Design review of the part built by this model. Coordinates are the model's own, in mm. A direction names the side the tool comes from. Coordinates: 2 decimals unless noted, no trailing zeros. Loops run counter-clockwise (first coordinate to the right, second up) from the corner with the lowest first, then second, coordinate; pieces in that order, holes last. Notation, with made-up numbers: (33, -2) - (90, -2) arc R34 ccw to (90, 35) - close; hole circle Ø10 at (-4.5, 35). An arc over 180 degrees is marked (long way). Use one line per item in the form item = value. Start each with the question number.
(1) For L1, parallel to Z at x = 0, y = -20; L2, parallel to Y at x = 31, z = 137.5; L3, parallel to Z at x = 0, y = -113.5, list the stretches that pass through material, from the lowest coordinate up.
(2) Clearance check with flat-ended pins moving along their axes: pin 1 Ø1.5 at (x, z) = (-20.5, 93.5) entering from +Y; pin 2 Ø5 at (x, y) = (36.5, -26.5) entering from +Z; pin 3 Ø10 at (y, z) = (-75, -24.5) entering from -X; pin 4 Ø20.5 at (y, z) = (-119, 65) entering from +X. State where each tip first meets the part, or that it passes through.
(3) Add section D-D (z = 34.5). State the section outline as (x, y) points.
(4) Tool access review of faces 1 (the face through (-9.97, -62.61, -44.9)), 2 (the face through (-45.142, -13, 59)), 3 (the face through (-0.993, -12.522, 155.356)): name each direction out of +Z, -Z, +X, -X, +Y, -Y from which nothing blocks a thin tool from reaching the whole face with its end or side.
(5) The part is to be moulded in two halves that separate along Z. For faces 4 (the face through (-3.374, -64.389, -15.192)), 5 (the face through (45.862, -114, 56)), 6 (the face through (3.25, -114.12, 119.93)), 7 (the face through (1.007, -114.478, 156.372)), say which applies: pulls with the +Z half, pulls with the -Z half, needs draft (parallel to the pull), parting line crosses it, or undercut.
(6) Add section A-A (x = 0). State the section outline as (y, z) points.
(7) Add section B-B (z = 66). State the section outline as (x, y) points.
(8) Add section C-C (y = -108.5). State the section outline as (x, z) points.
```python
from build123d import *

# Parameters (mm, degrees)
F0_R      = 45.9953933043
F1_DEPTH  = 127
F2_R      = 15.5126771319
F3_DEPTH  = 127
F4_W      = 91.7238295078
F4_H      = 110.3479489684
F5_DEPTH  = 25.4
F6_R      = 15.5623091615
F7_DEPTH  = 127
F8_R      = 45.8026969915
F9_DEPTH  = 25.4
F10_W     = 90.2835130692
F10_H     = 110.5170249939
F11_DEPTH = 25.4
F12_R     = 15.4559946756
F13_DEPTH = 127
F15_DEPTH = 25.4
F16_R     = 14.9850437789
F17_DEPTH = 127


with BuildPart() as f1:
    # F0 (on Front) → F1 (new body)
    with BuildSketch(Plane.XZ):
        Circle(F0_R)
    extrude(amount=F1_DEPTH)

    # F2 (on Front) → F3 (cut)
    with BuildSketch(Plane.XZ):
        Circle(F2_R)
    extrude(amount=F3_DEPTH, mode=Mode.SUBTRACT)

    # F4 (on face) → F5 (join)
    with BuildSketch(Plane.XZ.offset(127)):
        with Locations((0, 55.4068051279)):
            Rectangle(F4_W, F4_H)
    extrude(amount=-F5_DEPTH)

    # F6 (on face) → F7 (cut)
    with BuildSketch(Plane.XZ.offset(127)):
        Circle(F6_R)
    extrude(amount=-F7_DEPTH, mode=Mode.SUBTRACT)

    # F8 (on face) → F9 (join)
    with BuildSketch(Plane.XZ.offset(127)):
        with Locations((0, 110.5807796121)):
            Circle(F8_R)
    extrude(amount=-F9_DEPTH)

    # F10 (on face) → F11 (join)
    with BuildSketch(Plane(origin=(0, 0, 0), x_dir=(-1, 0, 0), z_dir=(0, 1, 0))):
        with Locations((0, 54.9663677812)):
            Rectangle(F10_W, F10_H)
    extrude(amount=-F11_DEPTH)

    # F12 (on face) → F13 (cut)
    with BuildSketch(Plane(origin=(0, 0, 0), x_dir=(-1, 0, 0), z_dir=(0, 1, 0))):
        Circle(F12_R)
    extrude(amount=-F13_DEPTH, mode=Mode.SUBTRACT)

    # F14 (on face) → F15 (join)
    with BuildSketch(Plane(origin=(0, 0, 0), x_dir=(-1, 0, 0), z_dir=(0, 1, 0))):
        with BuildLine():
            Line((-45.1417565346, 110.2248802781), (45.1417565346, 110.2248802781))
            ThreePointArc((45.1417565346, 110.2248802781), (0, 155.3666368127), (-45.1417565346, 110.2248802781))
        make_face()
    extrude(amount=-F15_DEPTH)

    # F16 (on face) → F17 (cut)
    with BuildSketch(Plane(origin=(0, 0, 0), x_dir=(-1, 0, 0), z_dir=(0, 1, 0))):
        with Locations((0, 134.5566511154)):
            Circle(F16_R)
    extrude(amount=-F17_DEPTH, mode=Mode.SUBTRACT)


solid = f1.part
```
Computed values:
q1.L1 = -46 to -15.56, 15.46 to 119.57, 149.54 to 155.37
q1.L2 = -127 to -101.6, -25.4 to 0
q1.L3 = -46 to -15.56, 15.56 to 119.57, 149.54 to 156.38
q2.pin_1 = 0
q2.pin_2 = 139.63
q2.pin_3 = -41.66
q2.pin_4 = 45.86
q3.outline = (-45.86, -127) - (45.86, -127) - (45.86, -101.6) - (30.42, -101.6) - (30.42, -25.4) - (45.14, -25.4) - (45.14, 0) - (-45.14, 0) - (-45.14, -25.4) - (-30.42, -25.4) - (-30.42, -101.6) - (-45.86, -101.6) - close
q4.face_1 = none
q4.face_2 = +Z, -X, +Y
q4.face_3 = +Z, +Y
q5.face_4 = undercut
q5.face_5 = needs draft
q5.face_6 = undercut
q5.face_7 = pulls with the +Z half
q6.outline = (-127, -46) - (0, -46) - (0, -15.56) - (-127, -15.56) - close; (-127, 15.56) - (-25.4, 15.56) - (-25.4, 15.46) - (0, 15.46) - (0, 119.57) - (-25.4, 119.57) - (-25.4, 46) - (-101.6, 46) - (-101.6, 119.57) - (-127, 119.57) - close; (-127, 149.54) - (-101.6, 149.54) - (-101.6, 156.38) - (-127, 156.38) - close; (-25.4, 149.54) - (0, 149.54) - (0, 155.37) - (-25.4, 155.37) - close
q7.outline = (-45.86, -127) - (45.86, -127) - (45.86, -101.6) - (-45.86, -101.6) - close; (-45.14, -25.4) - (45.14, -25.4) - (45.14, 0) - (-45.14, 0) - close
q8.outline = (-45.86, 3.5) arc R46 ccw (long way) to (45.86, 3.5) - (45.86, 110.58) - (45.8, 110.58) arc R45.8 ccw to (-45.8, 110.58) - (-45.86, 110.58) - close; hole circle Ø31.12 at (0, 0); hole circle Ø29.97 at (0, 134.56)
